For this review, take the finished solid that the model builds, in its own axes (mm). A direction names the side the tool comes from. Round coordinates to 2 decimals unless told otherwise and drop trailing zeros. Write each loop counter-clockwise with the first axis right and the second up, starting at its lowest first coordinate (ties: lowest second). Pieces come first, ordered by that corner, then holes. Notation, with made-up numbers: (-25, -28) -> (20, -28) arc R21 cw to (20, -16) -> close; hole circle Ø2 at (29.5, 86). An arc over 180 degrees is marked (long way). Answer in a Markdown table with one row per item. Add a question column.
```python
from build123d import *

# Parameters (mm, degrees)
SKETCH1_R           = 22.5
BOSS_EXTRUDE1_DEPTH = 15
SKETCH2_R           = 15
BOSS_EXTRUDE2_DEPTH = 102
SKETCH3_R           = 2.5
CUT_EXTRUDE1_DEPTH  = 51


with BuildPart() as part:
    # Sketch1 → Boss-Extrude1 (new body)
    with BuildSketch(Plane.XY):
        Circle(SKETCH1_R)
    extrude(amount=BOSS_EXTRUDE1_DEPTH)

    # Sketch2 → Boss-Extrude2 (add)
    with BuildSketch(Plane.XY.offset(15)):
        Circle(SKETCH2_R)
    extrude(amount=BOSS_EXTRUDE2_DEPTH)

    # Sketch3 → Cut-Extrude1 (cut, symmetric)
    with BuildSketch(Plane(origin=(0, 0, 0), x_dir=(1, 0, 0), z_dir=(0, 1, 0))):
        with Locations(Location((0, -102, 0), (0, 0, 270))):
            Circle(SKETCH3_R)
    extrude(amount=CUT_EXTRUDE1_DEPTH, both=True, mode=Mode.SUBTRACT)


solid = part.part
```
1. We need section A-A (x = 0). Write out the cut boundary in (y, z), plus the area to 4 significant figures.
2. Tool access review of faces 4 (the flat face through (15, -5, 15)), 5 (the flat face through (0, 0, 0)): name each direction out of +Z, -Z, +X, -X, +Y, -Y from which nothing blocks a thin tool from reaching the whole face with its end or side.
3. For L1, parallel to Z at x = 0, y = 7.5; L2, parallel to Z at x = 3.5, y = 19.5; L3, parallel to X at y = 8, z = 102, list the stretches that pass through material, from the lowest coordinate up. Write a range as [from, to].
4. The part is to be moulded in two halves that separate along X. For faces 1 (the flat face through (0, 0, 117)), 2 (the cylindrical face through (-14.985, 0.66, 65.286)), 3 (the cylindrical face through (0.751, 0.21, 104.385)), say which applies: pulls with the +X half, pulls with the -X half, needs draft (parallel to the pull), parting line crosses it, or undercut.
5. We need section C-C (z = 102). Write out the cut boundary in (x, y), plus the area to 3 significant figures.
6. Clearance check with flat-ended pins moving along their axes: pin 1 Ø12 at (x, z) = (-12.5, 60) entering from +Y; pin 2 Ø8 at (x, z) = (-1.5, 101.5) entering from +Y; pin 3 Ø1 at (x, z) = (-17, 64.5) entering from +Y; pin 4 Ø1.5 at (x, z) = (8, 74.5) entering from +Y. State where each tip first meets the part, or that it passes through.
7. We need section D-D (x = 10.5). Write out the cut boundary in (y, z), plus the area to 3 significant figures.
8. We need section B-B (y = 0). Write out the cut boundary in (x, z), plus the area to 3 significant figures.
Response:
| question | item | result |
|---|---|---|
| 1 | outline | (-22.5, 0) -> (22.5, 0) -> (22.5, 15) -> (15, 15) -> (15, 99.5) -> (-15, 99.5) -> (-15, 15) -> (-22.5, 15) -> close; (-15, 104.5) -> (15, 104.5) -> (15, 117) -> (-15, 117) -> close |
| 1 | area | 3,585 mm2 |
| 2 | face 4 | +Z |
| 2 | face 5 | -Z, +X, -X, +Y, -Y |
| 3 | L1 | [0, 99.5], [104.5, 117] |
| 3 | L2 | [0, 15] |
| 3 | L3 | [-12.69, -2.5], [2.5, 12.69] |
| 4 | face 1 | needs draft |
| 4 | face 2 | parting line crosses it |
| 4 | face 3 | undercut |
| 5 | outline | (-2.5, -14.79) -> (-2.5, 14.79) arc R15 ccw to start; (2.5, -14.79) arc R15 ccw to (2.5, 14.79) -> close |
| 5 | area | 558 mm2 |
| 6 | pin 1 | y = 13.52 |
| 6 | pin 2 | y = 15 |
| 6 | pin 3 | through |
| 6 | pin 4 | y = 13.13 |
| 7 | outline | (-19.9, 0) -> (19.9, 0) -> (19.9, 15) -> (10.71, 15) -> (10.71, 117) -> (-10.71, 117) -> (-10.71, 15) -> (-19.9, 15) -> close |
| 7 | area | 2,780 mm2 |
| 8 | outline | (-22.5, 0) -> (22.5, 0) -> (22.5, 15) -> (15, 15) -> (15, 117) -> (-15, 117) -> (-15, 15) -> (-22.5, 15) -> close; hole circle Ø5 at (0, 102) |
| 8 | area | 3,720 mm2 |
